Drawing for the job (mm, zero at the part's lowest x, y, z). A direction names the side the tool comes from. Round coordinates to 2 decimals unless told otherwise and drop trailing zeros. Order: outer loops, then holes, each group sorted by start corner. A loop starts at its lowest first (then second) coordinate and runs counter-clockwise, first axis right, second up. Notation, with made-up numbers: (33, 88.5) -> (75, 88.5) arc R22 ccw to (75, 99.5) -> close; hole circle Ø6 at (85, 11.5). An arc over 180 degrees is marked (long way). Use CSV: the item, a comma, the result in double quotes.
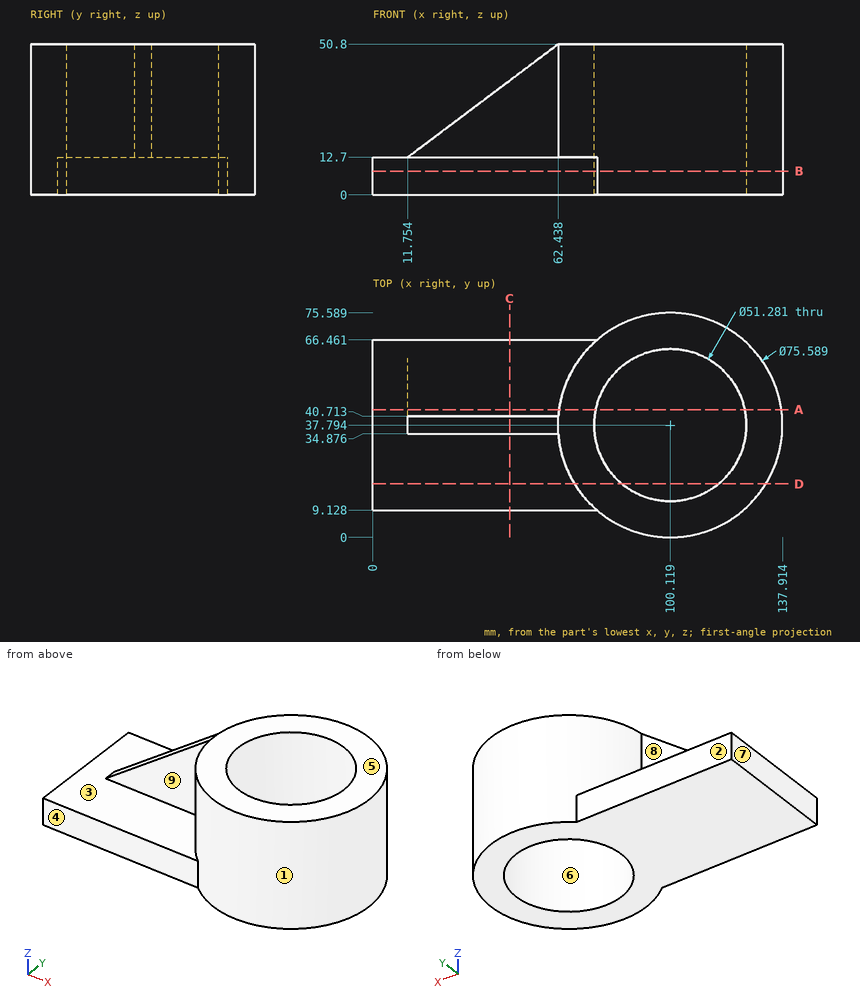
Q1. Probe line 1 along Y through (x, z) = (42.5, 33); line 2 along X through (y, z) = (32.5, 36.5); line 3 along Z through (x, y) = (14.5, 51). List the from-to ranges inside material, lowest first.
From the geometry:
line 1,"y = 34.88 to 40.71"
line 2,"x = 62.7 to 75.03, 125.21 to 137.54"
line 3,"z = 0 to 12.7"
Q2. Pin check, flat tips, straight feed: pin 1 (2 mm diameter, centred on y = 49.5, z = 22, fed in from +X); pin 2 (5 mm diameter, centred on y = 36, z = 15, fed in from +X); pin 3 (17 mm diameter, centred on x = 33, y = 38, fed in from +Z). Stop position of each tip, or through.
From the geometry:
pin 1,"stops at x = 136.37"
pin 2,"stops at x = 137.91"
pin 3,"stops at z = 35.06"
Q3. Mould opens along Y. For the marked faces 6, 7, 8 and 9 say: +Y half, -Y half, draft (parallel to the pull), parting line (faces both ways), or undercut.
From the geometry:
face 6,"undercut"
face 7,"draft"
face 8,"+Y half"
face 9,"-Y half"
Q4. Cut at B-B (z = 8). Give the cut face in (x, y) (1 decimal).
From the geometry:
outline,"(0, 9.1) -> (75.5, 9.1) arc R37.8 ccw (long way) to (75.5, 66.5) -> (0, 66.5) -> close; hole circle Ø51.3 at (100.1, 37.8)"
Q5. Cut at D-D (y = 18). Give the cut face in (x, z) (1 decimal).
From the geometry:
outline,"(0, 0) -> (83.8, 0) -> (83.8, 50.8) -> (67.9, 50.8) -> (67.9, 12.7) -> (0, 12.7) -> close; (116.4, 0) -> (132.3, 0) -> (132.3, 50.8) -> (116.4, 50.8) -> close"
Q6. Cut at A-A (y = 43). Give the cut face in (x, z) (1 decimal).
From the geometry:
outline,"(0, 0) -> (75, 0) -> (75, 50.8) -> (62.7, 50.8) -> (62.7, 12.7) -> (0, 12.7) -> close; (125.2, 0) -> (137.6, 0) -> (137.6, 50.8) -> (125.2, 50.8) -> close"
Q7. Cut at C-C (x = 46). Give the cut face in (y, z).
From the geometry:
outline,"(9.13, 0) -> (66.46, 0) -> (66.46, 12.7) -> (40.71, 12.7) -> (40.71, 38.44) -> (34.88, 38.44) -> (34.88, 12.7) -> (9.13, 12.7) -> close"
Q8. Which spindle directions (+Z, -Z, +X, -X, +Y, -Y) get a long thin tool onto all of the face, cutting with end or side? Do the marked faces 1, 2, 3, 4 and 5. Say none if no direction does.
From the geometry:
face 1,"+Z"
face 2,"+Z, -Z, -X, +Y"
face 3,"+Z, -X"
face 4,"+Z, -Z, -X, -Y"
face 5,"+Z, +X, -X, +Y, -Y"
